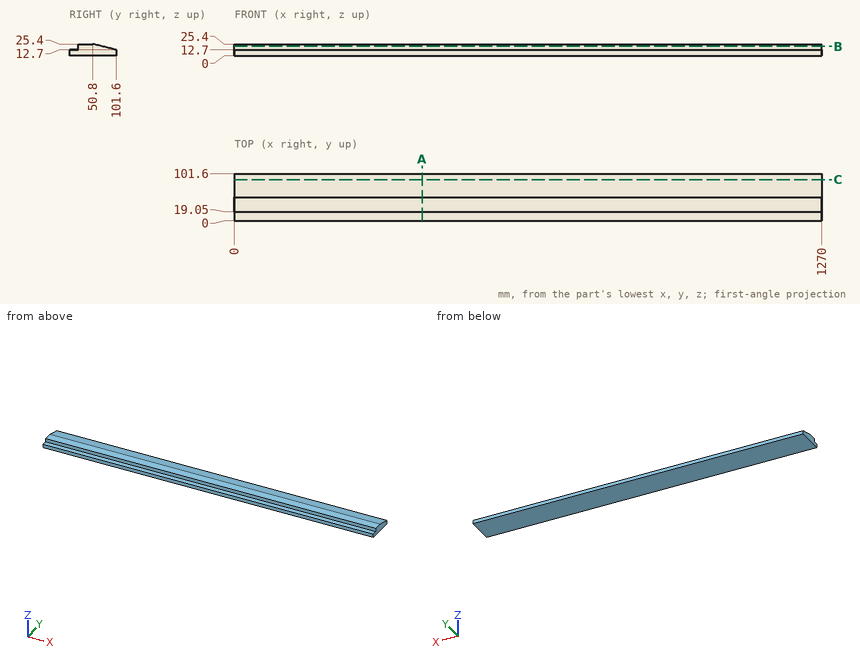
Source: three-view drawing plus pictorial views. Frame: mm from the lowest corner of the part. Round coordinates to 2 decimals unless told otherwise and drop trailing zeros. Loops run counter-clockwise (first coordinate to the right, second up) from the corner with the lowest first, then second, coordinate; pieces in that order, holes last.
1. Contact query for flat-ended pins moving along their axis: pin 1 (6.5 mm diameter, centred on x = 430.5, z = 19.5, fed in from -Y); pin 2 (5.5 mm diameter, centred on x = 841, y = 10, fed in from +Z); pin 3 (8 mm diameter, centred on x = 272.5, y = 60, fed in from +Z). Output: stop coordinate, or through.
2. Section query B-B on z = 20. Output: boundary loops of the cut face in (x, y).
3. Section query C-C on y = 89. Output: boundary loops of the cut face in (x, z).
4. Section query A-A on x = 406. Output: boundary loops of the cut face in (y, z), and give its area (3 significant figures).
5. Ray query, L1, parallel to Z at x = 58.5, y = 10; L2, parallel to Z at x = 1144.5, y = 57.5 (3 decimals). Return the intervals inside material, ascending.
Answers below:
1. pin 1: stops at y = 19.05
1. pin 2: stops at z = 12.7
1. pin 3: stops at z = 24.1
2. outline: (0, 19.05) - (1270, 19.05) - (1270, 72.4) - (0, 72.4) - close
3. outline: (0, 0) - (1270, 0) - (1270, 15.85) - (0, 15.85) - close
4. outline: (0, 0) - (101.6, 0) - (101.6, 12.7) - (50.8, 25.4) - (19.05, 25.4) - (19.05, 12.7) - (0, 12.7) - close
4. area: 2,020 mm2
5. L1: z = 0 to 12.7
5. L2: z = 0 to 23.725
